from build123d import *

# Parameters (mm, degrees)
SKETCH_1_W          = 93
SKETCH_1_H          = 20
EXTRUDE_1_DEPTH     = 1.5
SKETCH_2_W          = 93
SKETCH_2_H          = 20
SKETCH_2_W_2        = 89
SKETCH_2_H_2        = 17
EXTRUDE_2_DEPTH     = 20.5
SKETCH_3_W          = 14
SKETCH_3_H          = 1.5
CUT_EXTRUDE_1_DEPTH = 101.5
SKETCH_4_R          = 5.5
CUT_EXTRUDE_4_DEPTH = 3
EXTRUDE_3_DEPTH     = 3
SKETCH_7_W          = 3
SKETCH_7_H          = 17
CUT_EXTRUDE_6_DEPTH = 20.5


with BuildPart() as part:
    # Эскиз1 → Бобышка-Вытянуть1 (new body)
    with BuildSketch(Plane.XY):
        Rectangle(SKETCH_1_W, SKETCH_1_H)
    extrude(amount=EXTRUDE_1_DEPTH)

    # Эскиз2 → Бобышка-Вытянуть2 (add)
    with BuildSketch(Plane.XY.offset(1.5)):
        Rectangle(SKETCH_2_W, SKETCH_2_H)
        with Locations((-0.5, 0)):
            Rectangle(SKETCH_2_W_2, SKETCH_2_H_2, mode=Mode.SUBTRACT)
    extrude(amount=EXTRUDE_2_DEPTH)

    # Эскиз3 → Вырез-Вытянуть1 (cut)
    with BuildSketch(Plane(origin=(46.5, 0, 0), x_dir=(0, 0, -1), z_dir=(1, 0, 0))):
        with Locations((-15, -9.25)):
            Rectangle(SKETCH_3_W, SKETCH_3_H)
    extrude(amount=-CUT_EXTRUDE_1_DEPTH, mode=Mode.SUBTRACT)

    # Эскиз4 → Вырез-Вытянуть4 (cut)
    with BuildSketch(Plane(origin=(46.5, 0, 0), x_dir=(0, 0, -1), z_dir=(1, 0, 0))):
        with Locations((-13.5, 1.5)):
            Circle(SKETCH_4_R)
    extrude(amount=-CUT_EXTRUDE_4_DEPTH, mode=Mode.SUBTRACT)

    # Эскиз6 → Бобышка-Вытянуть3 (add)
    with BuildSketch(Plane.ZY.offset(46.5)):
        Polygon((0, 10), (22, 10), (22, -8.5), (8, -8.5), (8, -10), (0, -10), (0, -8.5), align=None)
    extrude(amount=EXTRUDE_3_DEPTH)

    # Эскиз7 → Вырез-Вытянуть6 (cut)
    with BuildSketch(Plane.XY.offset(22)):
        with Locations((-46.5, 0)):
            Rectangle(SKETCH_7_W, SKETCH_7_H)
    extrude(amount=-CUT_EXTRUDE_6_DEPTH, mode=Mode.SUBTRACT)


solid = part.part
Design review of the part built by this model. Coordinates are the model's own, in mm. A direction names the side the tool comes from. Round coordinates to 2 decimals unless told otherwise and drop trailing zeros. Write each loop counter-clockwise with the first axis right and the second up, starting at its lowest first coordinate (ties: lowest second). Pieces come first, ordered by that corner, then holes. Notation, with made-up numbers: (4.25, 34.25) - (37.25, 34.25) arc R5 ccw to (37.25, 41.25) - close; hole circle Ø2 at (66, 56.25). An arc over 180 degrees is marked (long way). Use a Markdown table: item, result. Add a question column.
1. Wall thickness on probe 1 along Y at (x, z) = (44.7, 13.5); probe 2 along X at (y, z) = (-8.25, 7); probe 3 along Z at (x, y) = (22.5, 5.75): over which ranges is each line inside the solid? List them lowest first.
2. For faces 1 (the face through (45, -8.5, 15)), 2 (the face through (-48, 0, 12)), 3 (the face through (-1, 0, 0)), list the 3-axis set-ups (+Z, -Z, +X, -X, +Y, -Y) from which the entire face can be reached by the end or side of a thin tool; tool diameter is ignored.
3. We need section C-C (y = 1.5). State the section outline as (x, z) points, then the cut area to 4 significant figures.
4. Mouldability with a two-part tool opening along Y and no side actions: class faces 4 (the face through (-1, -10, 4)), 5 (the face through (-3, 8.5, 12)), 6 (the face through (13, 9, 22)), 7 (the face through (45.268, 3.152, 8.254)) as +Y half, -Y half, draft (parallel to the pull), parting line (faces both ways), or undercut.
5. We need section B-B (z = 3.5). State the section outline as (x, y) points, then the cut area to 3 significant figures.
6. Clearance check with flat-ended pins moving along their axes: pin 1 (1.6 mm diameter, centred on x = 12, y = -9.5, fed in from +Z); pin 2 (1.2 mm diameter, centred on x = -48.5, z = 13.5, fed in from -Y); pin 3 (1.5 mm diameter, centred on x = 32, y = -0.5, fed in from +Z). State where each tip first meets the part, or that it passes through.
7. We need section A-A (z = 13.5). State the section outline as (x, y) points, then the cut area to 4 significant figures.
8. We need section D-D (x = 7). State the section outline as (y, z) points.
Output:
| question | item | result |
|---|---|---|
| 1 | probe 1 | y = -8.5 to -4, 7 to 10 |
| 1 | probe 2 | x = -49.5 to -48, 44 to 46.5 |
| 1 | probe 3 | z = 0 to 1.5 |
| 2 | face 1 | +Z, +X, -X, -Y |
| 2 | face 2 | +Z |
| 2 | face 3 | -Z, +X, -X, +Y, -Y |
| 3 | outline | (-49.5, 0) - (46.5, 0) - (46.5, 8) - (44, 8) - (44, 1.5) - (-48, 1.5) - (-48, 22) - (-49.5, 22) - close; (44, 19) - (46.5, 19) - (46.5, 22) - (44, 22) - close |
| 3 | area | 198.5 mm2 |
| 4 | face 4 | -Y half |
| 4 | face 5 | undercut |
| 4 | face 6 | draft |
| 4 | face 7 | undercut |
| 5 | outline | (-49.5, -10) - (46.5, -10) - (46.5, 10) - (-49.5, 10) - close; hole (-48, -8.5) - (44, -8.5) - (44, 8.5) - (-48, 8.5) - close |
| 5 | area | 356 mm2 |
| 6 | pin 1 | stops at z = 8 |
| 6 | pin 2 | stops at y = -8.5 |
| 6 | pin 3 | stops at z = 1.5 |
| 7 | outline | (-49.5, -8.5) - (-48, -8.5) - (-48, 8.5) - (44, 8.5) - (44, 7) - (46.5, 7) - (46.5, 10) - (-49.5, 10) - close; (44, -8.5) - (46.5, -8.5) - (46.5, -4) - (44, -4) - close |
| 7 | area | 184.5 mm2 |
| 8 | outline | (-10, 0) - (10, 0) - (10, 22) - (8.5, 22) - (8.5, 1.5) - (-8.5, 1.5) - (-8.5, 8) - (-10, 8) - close |
